Geometry: final body of the model. Coordinates: model frame, mm. A direction names the side the tool comes from. Give positions to 0.01 mm unless a question says otherwise; leave off trailing zeros. Write each loop counter-clockwise with the first axis right and the second up, starting at its lowest first coordinate (ties: lowest second). Pieces come first, ordered by that corner, then holes. Notation, with made-up numbers: M 27.5,29 L 49.5,29 A10 cw 49.5,40 Z; hole C 74.25,63.5 d2. An arc over 180 degrees is marked long. One line per question, with ' | ' between items.
from build123d import *

# Parameters (mm, degrees)
F0_W     = 30
F0_H     = 20
F1_DEPTH = 20
F3_DEPTH = 20.001
F4_DEPTH = 10
F5_DEPTH = 5


with BuildPart() as f1:
    # F0 (on Top) → F1 (new body)
    with BuildSketch(Plane.XY):
        with Locations((15, 10)):
            Rectangle(F0_W, F0_H)
    extrude(amount=F1_DEPTH)

    # F2 (on face) → F3 (cut, through all)
    with BuildSketch(Plane.XZ):
        with BuildLine():
            ThreePointArc((0.3175416345, 12.5), (3.876275643, 17.9056941504), (10, 20))
            Line((10, 20), (0, 20))
            Line((0, 20), (0, 10.0000000432))
            ThreePointArc((0, 10.0000000432), (0.07970304, 11.2600429462), (0.3175416345, 12.5))
        make_face()
        with BuildLine():
            ThreePointArc((0.3175416345, 7.5), (0.0797030346, 8.7399570966), (0, 10.0000000432))
            Line((0, 10.0000000432), (0, 0))
            Line((0, 0), (10, 0))
            ThreePointArc((10, 0), (3.876275643, 2.0943058496), (0.3175416345, 7.5))
        make_face()
        with BuildLine():
            ThreePointArc((15, 10), (14.8296291314, 11.2940952255), (14.3301270189, 12.5))
            ThreePointArc((14.3301270189, 12.5), (10, 15), (5.6698729811, 12.5))
            ThreePointArc((5.6698729811, 12.5), (5, 10), (5.6698729811, 7.5))
            ThreePointArc((5.6698729811, 7.5), (10, 5), (14.3301270189, 7.5))
            ThreePointArc((14.3301270189, 7.5), (14.8296291314, 8.7059047745), (15, 10))
        make_face()
        Polygon((30, 20), (25, 20), (30, 15), align=None)
        Polygon((30, 0), (30, 5), (25, 0), align=None)
    extrude(amount=-F3_DEPTH, mode=Mode.SUBTRACT)

    # F2 (on face) → F4 (cut)
    with BuildSketch(Plane.XZ):
        with BuildLine():
            Line((30, 7.5), (30, 12.5))
            Line((30, 12.5), (19.6824583655, 12.5))
            Line((19.6824583655, 12.5), (14.3301270189, 12.5))
            ThreePointArc((14.3301270189, 12.5), (14.8296291314, 11.2940952255), (15, 10))
            ThreePointArc((15, 10), (14.8296291314, 8.7059047745), (14.3301270189, 7.5))
            Line((14.3301270189, 7.5), (19.6824583655, 7.5))
            Line((19.6824583655, 7.5), (30, 7.5))
        make_face()
        with BuildLine():
            Line((5.6698729811, 12.5), (0.3175416345, 12.5))
            ThreePointArc((0.3175416345, 12.5), (0.07970304, 11.2600429462), (0, 10.0000000432))
            ThreePointArc((0, 10.0000000432), (0.0797030346, 8.7399570966), (0.3175416345, 7.5))
            Line((0.3175416345, 7.5), (5.6698729811, 7.5))
            ThreePointArc((5.6698729811, 7.5), (5, 10), (5.6698729811, 12.5))
        make_face()
    extrude(amount=-F4_DEPTH, mode=Mode.SUBTRACT)

    # F2 (on face) → F5 (cut)
    with BuildSketch(Plane.XZ):
        with BuildLine():
            Line((30, 5), (30, 7.5))
            Line((30, 7.5), (19.6824583655, 7.5))
            ThreePointArc((19.6824583655, 7.5), (16.123724357, 2.0943058496), (10, 0))
            Line((10, 0), (25, 0))
            Line((25, 0), (30, 5))
        make_face()
        with BuildLine():
            Line((30, 15), (25, 20))
            Line((25, 20), (10, 20))
            ThreePointArc((10, 20), (16.123724357, 17.9056941504), (19.6824583655, 12.5))
            Line((19.6824583655, 12.5), (30, 12.5))
            Line((30, 12.5), (30, 15))
        make_face()
    extrude(amount=-F5_DEPTH, mode=Mode.SUBTRACT)


solid = f1.part
(1) Cut plane D-D, the plane z = 13.5. Return loops of the section in (x, y), then the cut area to 3 significant figures.
Working result:
outline: M 0.63,0 L 6.43,0 L 6.43,20 L 0.63,20 Z; M 13.57,0 L 19.37,0 L 19.37,5 L 30,5 L 30,20 L 13.57,20 Z | area: 391 mm^2
(2) Cut plane A-A, the plane y = 3. Return loops of the section in (x, z).
Working result:
outline: M 0.32,7.5 A10 ccw 19.68,7.5 L 14.33,7.5 A5 cw 5.67,7.5 Z; M 0.32,12.5 L 5.67,12.5 A5 cw 14.33,12.5 L 19.68,12.5 A10 ccw Z
(3) Cut plane B-B, the plane x = 6. Return loops of the section in (y, z), then the cut area to 3 significant figures.
Working result:
outline: M 0,0.83 L 20,0.83 L 20,7 L 0,7 Z; M 0,13 L 20,13 L 20,19.17 L 0,19.17 Z | area: 247 mm^2
(4) Material intervals for L1, parallel to X at y = 19, z = 9.75; L2, parallel to Z at x = 21.75, y = 7; L3, parallel to X at y = 18, z = 7.5, sorted ascending. Write a range as [from, to].
Working result:
L1: x = [0, 5.01], [14.99, 30] | L2: z = [0, 7.5], [12.5, 20] | L3: x = [0.32, 5.67], [14.33, 30]
(5) Draft query along Z for faces 1 (the face through (22, 5, 4)), 2 (the face through (3, 10, 10)), 3 (the face through (17, 13, 20)). Return one class per face: released by +Z, released by -Z, zero draft, split by the parting line, or undercut.
Working result:
face 1: zero draft | face 2: undercut | face 3: released by +Z
(6) Set-up query: faces 4 (the face through (22, 5, 16)), 5 (the face through (30, 14, 10)), 6 (the face through (20, 6, 7.5)). Return all of +Z, -Z, +X, -X, +Y, -Y with unobstructed straight access to the full face (end or side cutting, diameter ignored); none if empty.
Working result:
face 4: +Z, +X, -Y | face 5: +Z, -Z, +X, +Y, -Y | face 6: +X, -X, -Y
(7) Cut plane C-C, the plane y = 13. Return loops of the section in (x, z).
Working result:
outline: M 10,0 L 25,0 L 30,5 L 30,15 L 25,20 L 10,20 A10 ccw Z; hole C 10,10 d10
(8) First-contact query: P1, Ø5, axis at x = 23, z = 3, coming from the -Y side; P2, Ø4.5, axis at x = 3.5, y = 5.5, coming from the +Z side; P3, Ø3, axis at x = 8, z = 8, coming from the +Y side; P4, Ø4.5, axis at x = 3.5, y = 5, coming from the -Z side. Flat tips, straight axial feed; report the tip coordinate or a pass-through.
Working result:
P1: stops at y = 5 | P2: stops at z = 19.05 | P3: passes through | P4: stops at z = 0.95
